For this review, use the dimensioned drawing (mm, ordinates from the lowest corner) and the shaded views. A direction names the side the tool comes from. Round coordinates to 2 decimals unless told otherwise and drop trailing zeros. Order: outer loops, then holes, each group sorted by start corner. A loop starts at its lowest first (then second) coordinate and runs counter-clockwise, first axis right, second up. Notation, with made-up numbers: M -10.75,-30 L 9.25,-30 A26 ccw 9.25,8 Z; hole C -5.5,29 d1. An arc over 180 degrees is marked long. Use a Markdown table: item, result. Add a question column.
1. To check wall thickness, follow probe 1 along Y at (x, z) = (40, 72.5); probe 2 along X at (y, z) = (63, 12); probe 3 along X at (y, z) = (57, 10). State the ranges of each line that lie inside material, in increasing order.
2. Consider section C-C on y = 47. State the section outline as (x, z) points, then the cut area to 3 significant figures.
3. For the marked faces 1, 2, 3 and 4, list the 3-axis set-ups (+Z, -Z, +X, -X, +Y, -Y) from which the entire face can be reached by the end or side of a thin tool; tool diameter is ignored.
4. Consider section A-A on z = 13. State the section outline as (x, y) points, then the cut area to 3 significant figures.
5. Consider section B-B on x = 40. State the section outline as (y, z) points.
6. Consider section D-D on z = 68.5. State the section outline as (x, y) points.
7. Insertion check: P1, Ø15, axis at y = 43.5, z = 68.5, coming from the -X side; P2, Ø1.5, axis at x = 60.5, y = 29, coming from the -Z side; P3, Ø15, axis at x = 38, y = 36, coming from the +Z side. Each pin has a flat end and moves straight along its axis. Give the tip position at first contact, or say it passes through.
8. The part is to be moulded in two halves that separate along Z. For the marked faces 5, 6 and 7, say which applies: +Z half, -Z half, draft (parallel to the pull), parting line (faces both ways), or undercut.
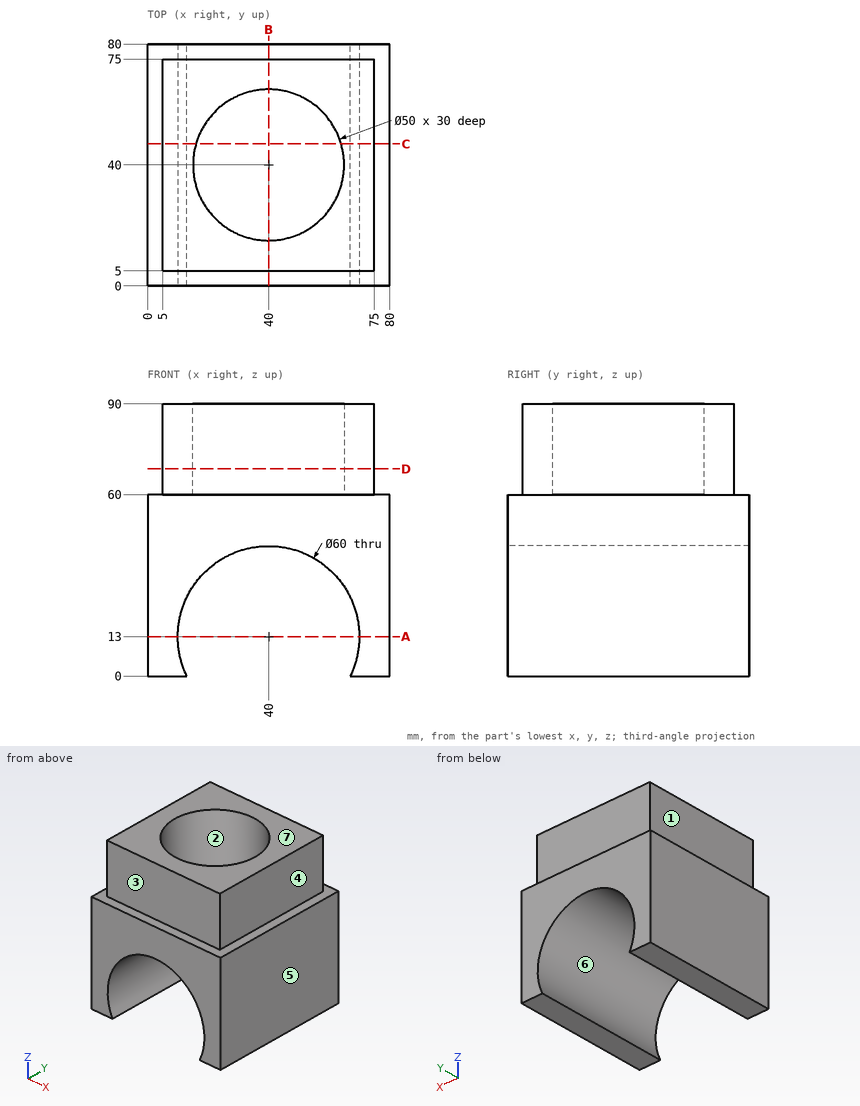
Answer block:
| question | item | result |
|---|---|---|
| 1 | probe 1 | 5 to 15, 65 to 75 |
| 1 | probe 2 | 0 to 10.02, 69.98 to 80 |
| 1 | probe 3 | 0 to 10.15, 69.85 to 80 |
| 2 | outline | M 0,0 L 12.96,0 A30 cw long 67.04,0 L 80,0 L 80,60 L 75,60 L 75,90 L 64,90 L 64,60 L 16,60 L 16,90 L 5,90 L 5,60 L 0,60 Z |
| 2 | area | 3,290 mm^2 |
| 3 | face 1 | +Z, -X, +Y, -Y |
| 3 | face 2 | +Z |
| 3 | face 3 | +Z, +X, -X, -Y |
| 3 | face 4 | +Z, +X, +Y, -Y |
| 4 | outline | M 0,0 L 10,0 L 10,80 L 0,80 Z; M 70,0 L 80,0 L 80,80 L 70,80 Z |
| 4 | area | 1,600 mm^2 |
| 5 | outline | M 0,43 L 80,43 L 80,60 L 75,60 L 75,90 L 65,90 L 65,60 L 15,60 L 15,90 L 5,90 L 5,60 L 0,60 Z |
| 6 | outline | M 5,5 L 75,5 L 75,75 L 5,75 Z; hole C 40,40 d50 |
| 7 | P1 | x = 5 |
| 7 | P2 | z = 34.18 |
| 7 | P3 | z = 60 |
| 8 | face 5 | draft |
| 8 | face 6 | undercut |
| 8 | face 7 | +Z half |
